from build123d import *

# Parameters (mm, degrees)
SKETCH1_W                            = 83.2
SKETCH1_H                            = 320
BOSS_EXTRUDE1_DEPTH                  = 1
F_3_0_3_DIAMETER_HOLE1_D             = 3
SKETCH_1_R                           = 11
CUT_EXTRUDE_1_DEPTH                  = 166.322593737
SKETCH_2_R                           = 6
CUT_EXTRUDE_2_DEPTH                  = 10
SKETCH_3_R                           = 1.5
CUT_EXTRUDE_3_DEPTH                  = 10
CHAMFER_1_SIZE                       = 1
PATTERN_CIRCULAR_1_COUNT             = 6
CHAMFER_1_OF_PATTERN_CIRCULAR_1_SIZE = 1
CUT_EXTRUDE_4_DEPTH                  = 10


with BuildPart() as part:
    # Sketch1 → Boss-Extrude1 (new body)
    with BuildSketch(Plane.XY):
        Rectangle(SKETCH1_W, SKETCH1_H)
    extrude(amount=BOSS_EXTRUDE1_DEPTH)

    # Ø3.0 (3) Diameter Hole1 (through all)
    with Locations(Plane.XY.offset(1)):
        with Locations((-30.5, 66), (30.5, 66), (30.5, -156), (-30.5, -156), (-30.5, 157.3), (30.5, 157.3), (-30.5, 47.3), (30.5, 47.3)):
            Hole(F_3_0_3_DIAMETER_HOLE1_D / 2)

    # Эскиз1 → Вырез-Вытянуть1 (cut, through all)
    with BuildSketch(Plane.XY.offset(1)):
        Circle(SKETCH_1_R)
    extrude(amount=-CUT_EXTRUDE_1_DEPTH, mode=Mode.SUBTRACT)

    # Эскиз2 → Вырез-Вытянуть2 (cut)
    with BuildSketch(Plane.XY.offset(1)):
        with Locations((0, -130)):
            Circle(SKETCH_2_R)
    extrude(amount=-CUT_EXTRUDE_2_DEPTH, mode=Mode.SUBTRACT)

    # Эскиз3 → Вырез-Вытянуть3 (cut)
    with BuildSketch(Plane.XY.offset(1)):
        with Locations((0, -120.5)):
            Circle(SKETCH_3_R)
    cut_extrude_3 = extrude(amount=-CUT_EXTRUDE_3_DEPTH, mode=Mode.SUBTRACT)

    # Фаска1
    chamfer_1_edges = [part.edges().sort_by_distance(p)[0] for p in [
        (-1.5, -120.5, 0),
    ]]
    chamfer(chamfer_1_edges, length=CHAMFER_1_SIZE - 0.0001)  # a hair under: the kernel refuses the full size

    # Круговой массив1: Вырез-Вытянуть3 ×6 about axis
    pattern_circular_1_axis = Axis((0, -130, 0), (0, 0, 1))
    for i in range(1, PATTERN_CIRCULAR_1_COUNT):
        add(cut_extrude_3.rotate(pattern_circular_1_axis, i * 360 / PATTERN_CIRCULAR_1_COUNT), mode=Mode.SUBTRACT)

    # Фаска1 of Круговой массив1
    chamfer_1_of_pattern_circular_1_edges = [part.edges().sort_by_distance(p)[0] for p in [
        (-8.977241336, -126.549038106, 0),
        (-7.477241336, -136.049038106, 0),
        (1.5, -139.5, 0),
        (8.977241336, -133.450961894, 0),
        (7.477241336, -123.950961894, 0),
    ]]
    chamfer(chamfer_1_of_pattern_circular_1_edges, length=CHAMFER_1_OF_PATTERN_CIRCULAR_1_SIZE - 0.0001)  # a hair under: the kernel refuses the full size

    # Эскиз4 → Вырез-Вытянуть4 (cut)
    with BuildSketch(Plane(origin=(0, 0, 0), x_dir=(-1, 0, 0), z_dir=(0, 0, -1))):
        with BuildLine():
            Line((-3.3, -100.29662602), (3.3, -100.29662602))
            ThreePointArc((3.3, -100.29662602), (4.219238816, -99.915864836), (4.6, -98.99662602))
            Line((4.6, -98.99662602), (4.6, -98.39662602))
            ThreePointArc((4.6, -98.39662602), (4.219238816, -97.477387205), (3.3, -97.09662602))
            Line((3.3, -97.09662602), (-3.3, -97.09662602))
            ThreePointArc((-3.3, -97.09662602), (-4.219238816, -97.477387205), (-4.6, -98.39662602))
            Line((-4.6, -98.39662602), (-4.6, -98.99662602))
            ThreePointArc((-4.6, -98.99662602), (-4.219238816, -99.915864836), (-3.3, -100.29662602))
        make_face()
    extrude(amount=-CUT_EXTRUDE_4_DEPTH, mode=Mode.SUBTRACT)


solid = part.part
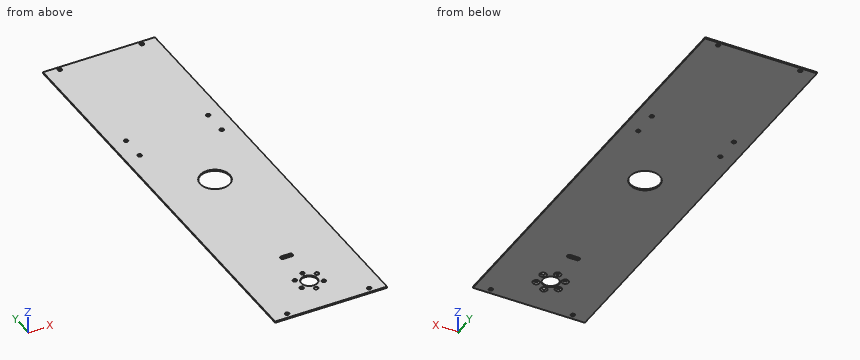
Can you work these out from the model? Positions are in its coordinate system, mm. Coordinates: 2 decimals unless noted, no trailing zeros. Loops run counter-clockwise (first coordinate to the right, second up) from the corner with the lowest first, then second, coordinate; pieces in that order, holes last. Notation, with made-up numbers: (-5, -40) - (16, -40) arc R34 ccw to (16, -4) - close; hole circle Ø10 at (81, 17). An arc over 180 degrees is marked (long way). Answer as a JSON object with one key per item and string values. Group by question number.
Item 1: If I drill on L1, parallel to Y at x = -30.5, z = 0.4; L2, parallel to X at y = 66, z = 0.6; L3, parallel to X at y = -133, z = 0.2, over which ranges is the centre line in solid material (lowest first)? Write a range as from..to.
Item 2: If we section it at A-A (y = 0): List the corners of the cut face in (x, z) for me, plus the area to 3 significant figures.
Item 3: If we section it at B-B (z = 0.35): State how many separate pieces and enclosed holes the cut face has, plus the area to 3 significant figures.
Item 4: For pin 1 (4 mm diameter, centred on x = -8.23, y = -125.25, fed in from -Z), with a flat end and sliding along its axis, tell me the tip position at first contact or that it passes through.
Returned:
{
 "1": {"L1": "y = -160..-157.5, -154.5..45.8, 48.8..64.5, 67.5..155.8, 158.8..160", "L2": "x = -41.6..-32, -29..29, 32..41.6", "L3": "x = -41.6..-9.72, -6.73..-5.2, 5.2..6.73, 9.72..41.6"},
 "2": {"outline": "(-41.6, 0) - (-11, 0) - (-11, 1) - (-41.6, 1) - close; (11, 0) - (41.6, 0) - (41.6, 1) - (11, 1) - close", "area": "61.2 mm²"},
 "3": {"separate pieces": "1", "enclosed holes": "17", "area": "26,000 mm²"},
 "4": {"pin 1": "stops at z = 0.5"}
}
